The model under review builds one solid part; all positions refer to its coordinate system, in mm. A direction names the side the tool comes from. Coordinates: 2 decimals unless noted, no trailing zeros. Write each loop counter-clockwise with the first axis right and the second up, starting at its lowest first coordinate (ties: lowest second). Pieces come first, ordered by that corner, then holes. Notation, with made-up numbers: M -7.5,-6 L 44.5,-6 A16 cw 44.5,20 Z; hole C 18,44.25 d1. An arc over 180 degrees is marked long. Answer as a JSON object with one key per item and string values.
```python
from build123d import *

# Parameters (mm, degrees)
F0_W        = 2
F0_H        = 2
F0_W_2      = 20
F0_H_2      = 3
F1_DEPTH    = 2
F2_T1_DEPTH = 12
F2_T3_DEPTH = 6.1421356237
F3_SIZE     = 0.1


# Not quite as in the source:
# - a fillet or chamfer that OpenCascade refuses, or shapes differently, is made with other operations: its cross-section is extruded or revolved along the edge and cut away or added


with BuildPart() as f1:
    # F0 (on Top) → F1 (new body)
    with BuildSketch(Plane.XY):
        with Locations((-11, 2.5)):
            Rectangle(F0_W, F0_H)
        with Locations((0, 2.5)):
            Rectangle(F0_W_2, F0_H)
        with Locations((11, 2.5)):
            Rectangle(F0_W, F0_H)
        with Locations((11, 0)):
            Rectangle(F0_W, F0_H_2)
        Polygon((12, -1.5), (10, -1.5), (11.4142135624, -2.9142135624), (12, -2.3284271247), align=None)
        Polygon((11.4142135624, -2.9142135624), (10, -1.5), (2.1213203436, -9.3786796564), (3.5355339059, -10.7928932188), align=None)
        with BuildLine():
            ThreePointArc((2.1213203436, -9.3786796564), (0, -10.2573593129), (-2.1213203436, -9.3786796564))
            Line((-2.1213203436, -9.3786796564), (-3.5355339059, -10.7928932188))
            ThreePointArc((-3.5355339059, -10.7928932188), (0, -12.2573593129), (3.5355339059, -10.7928932188))
            Line((3.5355339059, -10.7928932188), (2.1213203436, -9.3786796564))
        make_face()
        Polygon((-2.1213203436, -9.3786796564), (-10, -1.5), (-11.4142135624, -2.9142135624), (-3.5355339059, -10.7928932188), align=None)
        Polygon((-11.4142135624, -2.9142135624), (-10, -1.5), (-12, -1.5), (-12, -2.3284271247), align=None)
        with Locations((-11, 0)):
            Rectangle(F0_W, F0_H_2)
        with BuildLine():
            Line((0, -1.5), (-10, -1.5))
            Line((-10, -1.5), (-2.1213203436, -9.3786796564))
            ThreePointArc((-2.1213203436, -9.3786796564), (-1.1480502971, -4.4857207153), (3, -7.2573593129))
            ThreePointArc((3, -7.2573593129), (2.7716385975, -8.40540961), (2.1213203436, -9.3786796564))
            Line((2.1213203436, -9.3786796564), (10, -1.5))
            Line((10, -1.5), (0, -1.5))
        make_face()
    extrude(amount=F1_DEPTH)

    # F2: fillet of radius 2 on 4 edges, made by hand

    # F2_s2 → F2_t1 (cut)
    with BuildSketch(Plane.XY.offset(-5)):
        with BuildLine():
            ThreePointArc((-10, 3.5), (-11.4142135624, 2.9142135624), (-12, 1.5))
            Line((-12, 1.5), (-12, 3.5))
            Line((-12, 3.5), (-10, 3.5))
        make_face()
        with BuildLine():
            ThreePointArc((12, 1.5), (11.4142135624, 2.9142135624), (10, 3.5))
            Line((10, 3.5), (12, 3.5))
            Line((12, 3.5), (12, 1.5))
        make_face()
    extrude(amount=F2_T1_DEPTH, mode=Mode.SUBTRACT)

    # F2_s4 → F2_t3 (cut)
    with BuildSketch(Plane.XY.offset(-2.0710678119)):
        with BuildLine():
            ThreePointArc((-11.4142135624, -2.9142135624), (-11.847759065, -2.2653668647), (-12, -1.5))
            Line((-12, -1.5), (-12, -2.3284271247))
            Line((-12, -2.3284271247), (-11.4142135624, -2.9142135624))
        make_face()
        with BuildLine():
            ThreePointArc((11.4142135624, -2.9142135624), (11.847759065, -2.2653668647), (12, -1.5))
            Line((12, -1.5), (12, -2.3284271247))
            Line((12, -2.3284271247), (11.4142135624, -2.9142135624))
        make_face()
    extrude(amount=F2_T3_DEPTH, mode=Mode.SUBTRACT)

    # F3
    f3_edges = [f1.edges().sort_by_distance(p)[0] for p in [
        (-11.414214, 2.914214, 2),
        (0, 3.5, 2),
        (11.414214, 2.914214, 2),
        (12, 0, 2),
        (11.847759, -2.265367, 2),
        (7.474874, -6.853553, 2),
        (0, -12.257359, 2),
        (-7.474874, -6.853553, 2),
        (-11.847759, -2.265367, 2),
        (-12, 0, 2),
        (2.12132, -5.136039, 2),
        (0, 1.5, 2),
        (-10, 0, 2),
        (10, 0, 2),
        (0, -1.5, 2),
        (-11.414214, 2.914214, 0),
        (0, 3.5, 0),
        (11.414214, 2.914214, 0),
        (12, 0, 0),
        (11.847759, -2.265367, 0),
        (7.474874, -6.853553, 0),
        (0, -12.257359, 0),
        (-7.474874, -6.853553, 0),
        (-11.847759, -2.265367, 0),
        (-12, 0, 0),
        (2.12132, -5.136039, 0),
        (0, 1.5, 0),
        (-10, 0, 0),
        (10, 0, 0),
        (0, -1.5, 0),
    ]]
    chamfer(f3_edges, length=F3_SIZE)


solid = f1.part
```
(1) Add section C-C on x = 4.75. Give the boundary of the cut face in (y, z), and give its area (3 significant figures).
Results list:
{"outline": "M -9.58,0.1 L -9.44,0 L -1.6,0 L -1.5,0.1 L -1.5,1.9 L -1.6,2 L -9.44,2 L -9.58,1.9 Z; M 1.5,0.1 L 1.6,0 L 3.4,0 L 3.5,0.1 L 3.5,1.9 L 3.4,2 L 1.6,2 L 1.5,1.9 Z", "area": "20.1 mm²"}
(2) Add section D-D on x = -7.75. Give the boundary of the cut face in (y, z), and give its area (3 significant figures).
Results list:
{"outline": "M -6.58,0.1 L -6.44,0 L -1.6,0 L -1.5,0.1 L -1.5,1.9 L -1.6,2 L -6.44,2 L -6.58,1.9 Z; M 1.5,0.1 L 1.6,0 L 3.4,0 L 3.5,0.1 L 3.5,1.9 L 3.4,2 L 1.6,2 L 1.5,1.9 Z", "area": "14.1 mm²"}
(3) For faces 4 (the face through (10, 0, 1)), 5 (the face through (12, 0, 1)), list the 3-axis set-ups (+Z, -Z, +X, -X, +Y, -Y) from which the entire face can be reached by the end or side of a thin tool; tool diameter is ignored.
Results list:
{"face 4": "+Z, -Z", "face 5": "+Z, -Z, +X, +Y, -Y"}
(4) Add section A-A on x = 0. Give the boundary of the cut face in (y, z).
Results list:
{"outline": "M -12.26,0.1 L -12.16,0 L -10.36,0 L -10.26,0.1 L -10.26,1.9 L -10.36,2 L -12.16,2 L -12.26,1.9 Z; M -4.26,0.1 L -4.16,0 L -1.6,0 L -1.5,0.1 L -1.5,1.9 L -1.6,2 L -4.16,2 L -4.26,1.9 Z; M 1.5,0.1 L 1.6,0 L 3.4,0 L 3.5,0.1 L 3.5,1.9 L 3.4,2 L 1.6,2 L 1.5,1.9 Z"}
(5) Draft analysis for pull direction Y (two halves, no side actions). For faces 1 (the face through (-11.84, -2.28, 0.99)), 2 (the face through (0, -1.5, 1)), 3 (the face through (0, -3, 2)), state which applies: released by +Y, released by -Y, zero draft, split by the parting line, or undercut.
Results list:
{"face 1": "released by -Y", "face 2": "undercut", "face 3": "zero draft"}
(6) Add section B-B on z = 1.1. Give the boundary of the cut face in (x, y), and give its area (3 significant figures).
Results list:
{"outline": "M -12,-1.5 A2 ccw -11.41,-2.91 L -3.54,-10.79 A5 ccw 3.54,-10.79 L 11.41,-2.91 A2 ccw 12,-1.5 L 12,1.5 A2 ccw 10,3.5 L -10,3.5 A2 ccw -12,1.5 Z; hole M -10,-1.5 L 10,-1.5 L 10,1.5 L -10,1.5 Z; hole C 0,-7.26 d6", "area": "188 mm²"}
(7) Wall thickness on line 1 along Y through (x, z) = (0, 1.1); line 2 along X through (y, z) = (-0.75, 1.3); line 3 along Y through (x, z) = (-2.5, 0.4): over which ranges is each line inside the solid? List them lowest first. Write a range as from..to.
Results list:
{"line 1": "-12.26..-10.26, -4.26..-1.5, 1.5..3.5", "line 2": "-12..-10, 10..12", "line 3": "-11.59..-8.92, -5.6..-1.5, 1.5..3.5"}
